```python
from build123d import *

# Parameters (mm, degrees)
CROQUIS1_W              = 65.5
CROQUIS1_H              = 74
SALIENTE_EXTRUIR1_DEPTH = 1.8
CROQUIS2_W              = 5
CROQUIS2_H              = 74
SALIENTE_EXTRUIR2_DEPTH = 15
CROQUIS3_W              = 3.4
CROQUIS3_H              = 2.1
CORTAR_EXTRUIR1_DEPTH   = 74
SALIENTE_EXTRUIR4_DEPTH = 1.8
CROQUIS7_W              = 14
CROQUIS7_H              = 23
SALIENTE_EXTRUIR5_DEPTH = 3
CORTAR_EXTRUIR5_DEPTH   = 23
CROQUIS10_R             = 1
CORTAR_EXTRUIR6_DEPTH   = 8
CORTAR_EXTRUIR7_START   = -8
CROQUIS11_R             = 1
CORTAR_EXTRUIR7_DEPTH   = 8
CORTAR_EXTRUIR8_START   = -19.8
CROQUIS12_W             = 72.040317055
CROQUIS12_H             = 80.937811448
CROQUIS12_W_2           = 33.677278507
CROQUIS12_H_2           = 35.747817065
CORTAR_EXTRUIR8_DEPTH   = 16.8


with BuildPart() as part:
    # Croquis1 → Saliente-Extruir1 (new body)
    with BuildSketch(Plane.XY):
        with Locations((-58.211538462, -2.192307692)):
            Rectangle(CROQUIS1_W, CROQUIS1_H)
    extrude(amount=SALIENTE_EXTRUIR1_DEPTH)

    # Croquis2 → Saliente-Extruir2 (add)
    with BuildSketch(Plane.XY.offset(1.8)):
        with Locations((-88.461538462, -2.192307692)):
            Rectangle(CROQUIS2_W, CROQUIS2_H)
        with Locations((-27.961538462, -2.192307692)):
            Rectangle(CROQUIS2_W, CROQUIS2_H)
    extrude(amount=SALIENTE_EXTRUIR2_DEPTH)

    # Croquis3 → Cortar-Extruir1 (cut)
    with BuildSketch(Plane.XZ.offset(39.192307692)):
        Polygon((-88.461538462, 16.8), (-89.111538462, 16.8), (-89.111538462, 15.9), (-87.811538462, 15.9), (-87.811538462, 16.8), align=None)
        with Locations((-87.661538462, 13.95)):
            Rectangle(CROQUIS3_W, CROQUIS3_H)
        with Locations((-28.761538462, 13.95)):
            Rectangle(CROQUIS3_W, CROQUIS3_H)
        Polygon((-28.611538462, 16.8), (-27.961538462, 16.8), (-27.311538462, 16.8), (-27.311538462, 15.9), (-28.611538462, 15.9), align=None)
    extrude(amount=-CORTAR_EXTRUIR1_DEPTH, mode=Mode.SUBTRACT)

    # Croquis6 → Saliente-Extruir4 (add)
    with BuildSketch(Plane.XZ.offset(39.192307692)):
        Polygon((-85.961538462, 8.7), (-80.961538462, 8.7), (-80.961538462, 1.8), (-45.461538462, 1.8), (-45.461538462, 5.7), (-30.461538462, 5.7), (-25.461538462, 5.7), (-25.461538462, 0), (-90.961538462, 0), (-90.961538462, 8.7), align=None)
    extrude(amount=SALIENTE_EXTRUIR4_DEPTH)

    # Croquis7 → Saliente-Extruir5 (add)
    with BuildSketch(Plane(origin=(0, 0, 0), x_dir=(-1, 0, 0), z_dir=(0, 0, -1))):
        with Locations((58.211538462, -3.092307692)):
            Rectangle(CROQUIS7_W, CROQUIS7_H)
    extrude(amount=SALIENTE_EXTRUIR5_DEPTH)

    # Croquis9 → Cortar-Extruir5 (cut)
    with BuildSketch(Plane.XZ.offset(14.592307692)):
        Polygon((-51.211538462, -3), (-54.211538462, 0), (-51.211538462, 0), align=None)
        Polygon((-65.211538462, -3), (-62.211538462, 0), (-65.211538462, 0), align=None)
    extrude(amount=-CORTAR_EXTRUIR5_DEPTH, mode=Mode.SUBTRACT)

    # Croquis10 → Cortar-Extruir6 (cut)
    with BuildSketch(Plane.XZ.offset(39.192307692)):
        with Locations(Location((-87.661538462, 10.9, 0), (0, 0, 270))):
            Circle(CROQUIS10_R)
        with Locations(Location((-28.761538462, 10.9, 0), (0, 0, 270))):
            Circle(CROQUIS10_R)
    extrude(amount=-CORTAR_EXTRUIR6_DEPTH, mode=Mode.SUBTRACT)

    # Croquis11 → Cortar-Extruir7 (cut)
    with BuildSketch(Plane(origin=(0, 34.807692308, 0), x_dir=(1, 0, 0), z_dir=(0, 1, 0)).offset(CORTAR_EXTRUIR7_START)):
        with Locations(Location((-28.761538462, -10.9, 0), (0, 0, 90))):
            Circle(CROQUIS11_R)
        with Locations(Location((-87.661538462, -10.9, 0), (0, 0, 90))):
            Circle(CROQUIS11_R)
    extrude(amount=CORTAR_EXTRUIR7_DEPTH, mode=Mode.SUBTRACT)

    # Croquis12 → Cortar-Extruir8 (cut)
    with BuildSketch(Plane(origin=(0, 0, -3), x_dir=(-1, 0, 0), z_dir=(0, 0, -1)).offset(CORTAR_EXTRUIR8_START)):
        with Locations((57.367684443, -4.300620435)):
            Rectangle(CROQUIS12_W, CROQUIS12_H)
        with Locations((57.760041523, -1.524971817)):
            Rectangle(CROQUIS12_W_2, CROQUIS12_H_2, mode=Mode.SUBTRACT)
    extrude(amount=CORTAR_EXTRUIR8_DEPTH, mode=Mode.SUBTRACT)


solid = part.part
```
CAD build for the part. Positions are in the model's coordinates, mm. A direction names the side the tool comes from. Round coordinates to 2 decimals unless told otherwise and drop trailing zeros. Order: outer loops, then holes, each group sorted by start corner. A loop starts at its lowest first (then second) coordinate and runs counter-clockwise, first axis right, second up.
Item 1: Saw through at A-A on y = -13.5. Write the cut outline in (x, z), then the cut area to 3 significant figures.
Item 2: Saw through at B-B on x = -58.5. Write the cut outline in (y, z).
Item 3: Probe line 1 along Z through (x, y) = (-71, -0.5); line 2 along Y through (x, z) = (-63, -1.7); line 3 along Z through (x, y) = (-53, 0). List the from-to ranges inside material, lowest first.
Item 4: Saw through at D-D on z = -2.25. Write the cut outline in (x, y).
Item 5: Saw through at C-C on x = -63. Write the cut outline in (y, z), then the cut area to 3 significant figures.
Item 6: Tool access for faces 1 (the face through (-58, -14.592, -1)), 2 (the face through (-58, -19.399, 1)), 3 (the face through (-58, 8.408, -1)), 4 (the face through (-52.69, -3.25, -1.52)): list every direction of +Z, -Z, +X, -X, +Y, -Y with a clear straight run to the whole face (end or side of a thin tool).
Item 7: Mould opens along Z. For faces 5 (the face through (-58, 16.349, 1)), 6 (the face through (-58, -1, 1.8)), 7 (the face through (-63.73, -3.25, -1.52)) say: pulls with the +Z half, pulls with the -Z half, needs draft (parallel to the pull), parting line crosses it, or undercut.
Item 8: Pin check, flat tip, straight feed: pin 1 (1.5 mm diameter, centred on y = -5, z = -2.5, fed in from -X). Stop position of the tip, or through.
Reported:
1. outline: (-74.6, 0) - (-62.21, 0) - (-65.21, -3) - (-51.21, -3) - (-54.21, 0) - (-40.92, 0) - (-40.92, 1.8) - (-74.6, 1.8) - close
1. area: 93.6 mm2
2. outline: (-19.4, 0) - (-14.59, 0) - (-14.59, -3) - (8.41, -3) - (8.41, 0) - (16.35, 0) - (16.35, 1.8) - (-19.4, 1.8) - close
3. line 1: z = 0 to 1.8
3. line 2: y = -14.59 to 8.41
3. line 3: z = -3 to -1.21, 0 to 1.8
4. outline: (-64.46, -14.59) - (-51.96, -14.59) - (-51.96, 8.41) - (-64.46, 8.41) - close
5. outline: (-19.4, 0) - (16.35, 0) - (16.35, 1.8) - (-19.4, 1.8) - close; (-14.59, -3) - (8.41, -3) - (8.41, -0.79) - (-14.59, -0.79) - close
5. area: 115 mm2
6. face 1: -Z, +X, -X, -Y
6. face 2: +Z, -Z, +X, -X, -Y
6. face 3: -Z, +X, -X, +Y
6. face 4: +X, +Y, -Y
7. face 5: needs draft
7. face 6: pulls with the +Z half
7. face 7: undercut
8. pin 1: stops at x = -65.21
